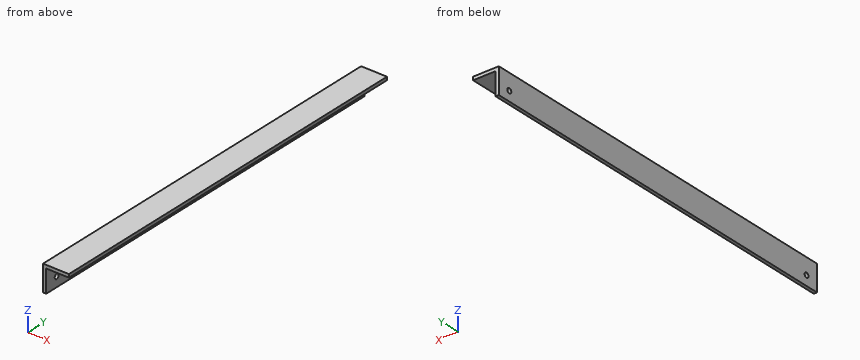
```python
from build123d import *

# Parameters (mm, degrees)
F1_DEPTH = 387.35
F2_R     = 2.38125
F3_DEPTH = 3.175


with BuildPart() as f1:
    # F0 (on Front) → F1 (new body)
    with BuildSketch(Plane.XZ):
        Polygon((0, 25.4), (0, 0), (3.175, 0), (3.175, 22.225), (25.4, 22.225), (25.4, 25.4), align=None)
    extrude(amount=-F1_DEPTH)

    # F2 (on face) → F3 (cut)
    with BuildSketch(Plane(origin=(0, 0, 0), x_dir=(0, -1, 0), z_dir=(-1, 0, 0))):
        with Locations((-12.7, 9.525)):
            Circle(F2_R)
        with Locations((-374.65, 9.525)):
            Circle(F2_R)
    extrude(amount=-F3_DEPTH, mode=Mode.SUBTRACT)


solid = f1.part
```
Source: CAD feature listing. Evaluate the final solid. Frame: model axes, mm. Give positions to 0.01 mm unless a question says otherwise; leave off trailing zeros. Loops run counter-clockwise (first coordinate to the right, second up) from the corner with the lowest first, then second, coordinate; pieces in that order, holes last. Notation, with made-up numbers: (-19, 13.5) -> (21, 13.5) arc R28 ccw to (21, 31.5) -> close; hole circle Ø8 at (87, 57). An arc over 180 degrees is marked (long way). Put each result on its own line as item: value. Start each with the question number.
1) Cut plane A-A (y = 120). Return loops of the section in (x, z) (3 decimals).
2) Cut plane B-B (x = 7.75). Return loops of the section in (y, z) (3 decimals), then the cut area to 3 significant figures.
3) Material intervals for probe 1 along Z at (x, y) = (2.2, 374.65); probe 2 along Z at (x, y) = (15.5, 238) (3 decimals); probe 3 along X at (y, z) = (206.5, 5.25) (3 decimals), sorted ascending.
4) Contact query for flat-ended pins moving along their axis: P1, Ø7.5, axis at y = 374.65, z = 9.525, coming from the +X side (3 decimals); P2, Ø6, axis at x = 20, y = 255.5, coming from the -Z side (3 decimals); P3, Ø4.5, axis at y = 12.7, z = 9.525, coming from the +X side. Output: stop coordinate, or through.
Results are:
1. outline: (0, 0) -> (3.175, 0) -> (3.175, 22.225) -> (25.4, 22.225) -> (25.4, 25.4) -> (0, 25.4) -> close
2. outline: (0, 22.225) -> (387.35, 22.225) -> (387.35, 25.4) -> (0, 25.4) -> close
2. area: 1,230 mm2
3. probe 1: z = 0 to 7.14, 11.91 to 25.4
3. probe 2: z = 22.225 to 25.4
3. probe 3: x = 0 to 3.175
4. P1: stops at x = 3.175
4. P2: stops at z = 22.225
4. P3: passes through
